from build123d import *


with BuildPart() as part:
    # Sketch1 → Revolve1 (revolve)
    with BuildSketch(Plane.XY):
        with BuildLine():
            Line((-20, 42.86), (7.886601718, 14.973398282))
            ThreePointArc((7.886601718, 14.973398282), (14.610917759, 11.091112606), (22.375489112, 11.091112606))
            Line((22.375489112, 11.091112606), (68.779388603, 23.525))
            Line((68.779388603, 23.525), (68.779388603, 26))
            Line((68.779388603, 26), (11, 26))
            Line((11, 26), (11, 35))
            Line((11, 35), (6, 35))
            Line((6, 35), (6, 33))
            Line((6, 33), (0, 33))
            Line((0, 33), (0, 42.86))
            Line((0, 42.86), (-20, 42.86))
        make_face()
    revolve(axis=Axis((0, 0, 0), (-1, 0, 0)))


solid = part.part
The listing builds one solid part. Answer for the finished solid, in the listing's coordinates (mm). A direction names the side the tool comes from. Coordinates: 2 decimals unless noted, no trailing zeros. Write each loop counter-clockwise with the first axis right and the second up, starting at its lowest first coordinate (ties: lowest second). Pieces come first, ordered by that corner, then holes. Notation, with made-up numbers: (69, 23) - (127, 23) arc R30 cw to (127, 48) - close; hole circle Ø7 at (-11.75, -11.5). An arc over 180 degrees is marked (long way). Answer as CSV lines item,"result".
1. Find section A-A (z = 0). Give the vertices of the cut face in (x, y) (3 decimals), plus the area to 3 significant figures.
Computed values:
outline,"(-20, -42.86) - (0, -42.86) - (0, -33) - (6, -33) - (6, -35) - (11, -35) - (11, -26) - (68.779, -26) - (68.779, -23.525) - (22.375, -11.091) arc R15 ccw to (7.887, -14.973) - close; (-20, 42.86) - (7.887, 14.973) arc R15 ccw to (22.375, 11.091) - (68.779, 23.525) - (68.779, 26) - (11, 26) - (11, 35) - (6, 35) - (6, 33) - (0, 33) - (0, 42.86) - close"
area,"1,910 mm²"
2. Find section C-C (x = 47.5). Give the vertices of the cut face in (y, z), plus the area to 3 significant figures.
Computed values:
outline,"circle Ø52 at (0, 0); hole circle Ø35.65 at (0, 0)"
area,"1,130 mm²"
3. Given P1, Ø1.5, axis at y = -28, z = -16.5, coming from the +X side; P2, Ø12, axis at x = 24, z = -26, coming from the +Y side; P3, Ø1.5, axis at x = 0, y = -13.5, coming from the -Z side; P4, Ø21, axis at y = 10.5, z = 14.5, coming from the +X side, each flat-ended and moving along its own axis, determine where each tip first touches the part or whether it passes through.
Computed values:
P1,"stops at x = 11"
P2,"stops at y = 16.61"
P3,"stops at z = -40.92"
P4,"stops at x = 68.78"
4. Straight lines are drawn through the part: line 1 (Z direction, x = -9.5, y = -13); line 2 (Y direction, x = 32, z = 9); line 3 (Y direction, x = -11, z = -15). For each, find the intervals that lie inside material, in ascending order. Write a range as [from, to].
Computed values:
line 1,"z = [-40.84, -29.63], [29.63, 40.84]"
line 2,"y = [-24.39, -10.29], [10.29, 24.39]"
line 3,"y = [-40.15, -30.36], [30.36, 40.15]"
5. Find section D-D (x = 57). Give the vertices of the cut face in (y, z), plus the area to 3 significant figures.
Computed values:
outline,"circle Ø52 at (0, 0); hole circle Ø40.74 at (0, 0)"
area,"820 mm²"
6. Determine the mould class of faces 3 (the cylindrical face through (3, 30.5, 12.6)), 4 (the cylindrical face through (-10.14, -34.01, 26.08)), 5 (the conical face through (6.533, 15.573, -4.904)), 6 (the flat face through (68.779, 6, 23)) for opening direction X: +X half, -X half, draft (parallel to the pull), parting line (faces both ways), or undercut.
Computed values:
face 3,"undercut"
face 4,"draft"
face 5,"-X half"
face 6,"+X half"
7. A tool of negligible diameter and unlimited length cuts with its end or side. For faces 1 (the flat face through (0, -22, 25)), 2 (the flat face through (11, 26.1, 2.4)), from which of +Z, -Z, +X, -X, +Y, -Y can it reach the whole face along a straight path? Write none if from no direction.
Computed values:
face 1,"none"
face 2,"+X"
